Could you check a few things on this model? Use its own coordinates, in mm. Face numbers are marked on the shaded views. A direction names the side the tool comes from. Give positions to 0.01 mm unless a question says otherwise; leave off trailing zeros. Loops run counter-clockwise (first coordinate to the right, second up) from the corner with the lowest first, then second, coordinate; pieces in that order, holes last. Notation, with made-up numbers: M -37,69 L 2,69 A28 ccw 2,91 Z; hole C -3,55 d11. An arc over 180 degrees is marked long. Use a Markdown table: item, result. Add a question column.
1) If I drill on line 1 along Y through (x, z) = (15.25, 3.5); line 2 along Y through (x, z) = (-14.15, 3.5); line 3 along Z through (x, y) = (-14.75, 5.5), over which ranges is the centre line in solid material (lowest first)? Write a range as [from, to].
2) Which directions (+Z, -Z, +X, -X, +Y, -Y) give clear straight access to the entire face, cutting with the end or side of a thin tool? Please do the marked faces 4, 5 and 6.
3) Suppose I cut it at A-A on x = 7. List the corners of the cut face in (y, z) for me, and give its area (3 significant figures).
4) We'd pull the mould along Y, two halves only. Please class the marked faces 1, 2 and 3: +Y half, -Y half, draft (parallel to the pull), parting line (faces both ways), or undercut.
5) Will these pins go through, and if not, where does the flat tip stop? pin 1 Ø1.8 at (y, z) = (-5.5, 3.5) entering from +X; pin 2 Ø3 at (x, y) = (-14.5, -4.5) entering from +Z; pin 3 Ø1.5 at (x, z) = (12.5, 5) entering from -Y.
6) Suppose I cut it at B-B on z = 5.5. List the corners of the cut face in (x, y) for me.
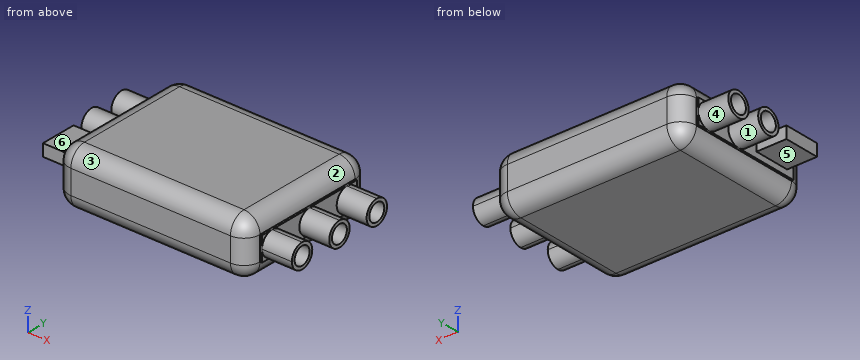
```python
from build123d import *

# Parameters (mm, degrees)
F1_DEPTH  = 7
F2_R      = 2
F3_R      = 1.1
F4_DEPTH  = 4
F5_R      = 1.5
F5_R_2    = 1.1
F6_DEPTH  = 4
F5_W      = 4.5
F5_H      = 1.5
F7_W      = 14
F7_H      = 3
F8_DEPTH  = 0.25
F9_W      = 14
F9_H      = 3
F10_DEPTH = 0.25


with BuildPart() as f1:
    # F0 (on Top) → F1 (new body)
    with BuildSketch(Plane.XY):
        with BuildLine():
            ThreePointArc((12, 7), (11.4142135624, 8.4142135624), (10, 9))
            Line((10, 9), (-10, 9))
            ThreePointArc((-10, 9), (-11.4142135624, 8.4142135624), (-12, 7))
            Line((-12, 7), (-12, -7))
            ThreePointArc((-12, -7), (-11.4142135624, -8.4142135624), (-10, -9))
            Line((-10, -9), (10, -9))
            ThreePointArc((10, -9), (11.4142135624, -8.4142135624), (12, -7))
            Line((12, -7), (12, 7))
        make_face()
    extrude(amount=F1_DEPTH)

    # F2
    f2_edges = [f1.edges().sort_by_distance(p)[0] for p in [
        (11.414214, 8.414214, 7),
        (0, 9, 7),
        (-11.414214, 8.414214, 7),
        (-12, 0, 7),
        (-11.414214, -8.414214, 7),
        (0, -9, 7),
        (11.414214, -8.414214, 7),
        (12, 0, 7),
        (11.414214, 8.414214, 0),
        (0, 9, 0),
        (-11.414214, 8.414214, 0),
        (-12, 0, 0),
        (-11.414214, -8.414214, 0),
        (0, -9, 0),
        (11.414214, -8.414214, 0),
        (12, 0, 0),
    ]]
    fillet(f2_edges, radius=F2_R)



with BuildPart() as f4:
    # F3 (on face) → F4 (new body)
    with BuildSketch(Plane.YZ.offset(12)):
        with BuildLine():
            ThreePointArc((-4, 3.5), (-4.4393398246, 4.5606601681), (-5.4999999897, 5))
            ThreePointArc((-5.4999999897, 5), (-6.5606601681, 4.5606601754), (-7, 3.5))
            ThreePointArc((-7, 3.5), (-6.5606601718, 2.4393398282), (-5.5, 2))
            ThreePointArc((-5.5, 2), (-4.4393398282, 2.4393398282), (-4, 3.5))
        make_face()
        with Locations((-5.5, 3.5)):
            Circle(F3_R, mode=Mode.SUBTRACT)
    extrude(amount=F4_DEPTH)


with BuildPart() as f4b:
    # F3 (on face) → F4, piece 2 (new body)
    with BuildSketch(Plane.YZ.offset(12)):
        with BuildLine():
            ThreePointArc((0, 2), (1.0606601718, 2.4393398282), (1.5, 3.5))
            ThreePointArc((1.5, 3.5), (1.0606601718, 4.5606601718), (0, 5))
            ThreePointArc((0, 5), (-1.5, 3.5), (0, 2))
        make_face()
        with Locations((0, 3.5)):
            Circle(F3_R, mode=Mode.SUBTRACT)
    extrude(amount=F4_DEPTH)


with BuildPart() as f4c:
    # F3 (on face) → F4, piece 3 (new body)
    with BuildSketch(Plane.YZ.offset(12)):
        with BuildLine():
            ThreePointArc((7, 3.5), (6.5606601718, 4.5606601718), (5.5, 5))
            ThreePointArc((5.5, 5), (4, 3.499999998), (5.5000000039, 2))
            ThreePointArc((5.5000000039, 2), (6.5606601732, 2.4393398296), (7, 3.5))
        make_face()
        with Locations((5.5, 3.5)):
            Circle(F3_R, mode=Mode.SUBTRACT)
    extrude(amount=F4_DEPTH)


with BuildPart() as f6:
    # F5 (on face) → F6 (new body)
    with BuildSketch(Plane(origin=(-12, 0, 0), x_dir=(0, -1, 0), z_dir=(-1, 0, 0))):
        with Locations((-5.5, 3.5)):
            Circle(F5_R)
        with Locations((-5.5, 3.5)):
            Circle(F5_R_2, mode=Mode.SUBTRACT)
    extrude(amount=F6_DEPTH)


with BuildPart() as f6b:
    # F5 (on face) → F6, piece 2 (new body)
    with BuildSketch(Plane(origin=(-12, 0, 0), x_dir=(0, -1, 0), z_dir=(-1, 0, 0))):
        with Locations((-1.1, 3.5)):
            Circle(F5_R)
        with Locations((-1.1, 3.5)):
            Circle(F5_R_2, mode=Mode.SUBTRACT)
    extrude(amount=F6_DEPTH)


with BuildPart() as f6c:
    # F5 (on face) → F6, piece 3 (new body)
    with BuildSketch(Plane(origin=(-12, 0, 0), x_dir=(0, -1, 0), z_dir=(-1, 0, 0))):
        with Locations((3.8085386623, 3.5)):
            Rectangle(F5_W, F5_H)
    extrude(amount=F6_DEPTH)


with BuildPart() as f1_1:
    add(f1.part)

    add(f4.part)  # F8 merges F4

    add(f4b.part)  # F8 merges F4b

    add(f4c.part)  # F8 merges F4c
    # F7 (on face) → F8 (join)
    with BuildSketch(Plane.YZ.offset(12)):
        with Locations((0, 3.5)):
            Rectangle(F7_W, F7_H)
    extrude(amount=F8_DEPTH)


    add(f6.part)  # F10 merges F6

    add(f6b.part)  # F10 merges F6b

    add(f6c.part)  # F10 merges F6c
    # F9 (on face) → F10 (join)
    with BuildSketch(Plane(origin=(-12, 0, 0), x_dir=(0, -1, 0), z_dir=(-1, 0, 0))):
        with Locations((0, 3.5)):
            Rectangle(F9_W, F9_H)
    extrude(amount=F10_DEPTH)


solid = f1_1.part
```
Answer block:
| question | item | result |
|---|---|---|
| 1 | line 1 | y = [-7, -6.6], [-4.4, -4], [-1.5, -1.1], [1.1, 1.5], [4, 4.4], [6.6, 7] |
| 1 | line 2 | y = [-6.06, -1.56], [-0.4, 0], [2.2, 2.6], [4, 4.4], [6.6, 7] |
| 1 | line 3 | z = [2, 2.4], [4.6, 5] |
| 2 | face 4 | -X |
| 2 | face 5 | -Z, -X, -Y |
| 2 | face 6 | +Z, -X, -Y |
| 3 | outline | M -9,2 A2 ccw -7,0 L 7,0 A2 ccw 9,2 L 9,5 A2 ccw 7,7 L -7,7 A2 ccw -9,5 Z |
| 3 | area | 123 mm^2 |
| 4 | face 1 | undercut |
| 4 | face 2 | draft |
| 4 | face 3 | -Y half |
| 5 | pin 1 | stops at x = 12.25 |
| 5 | pin 2 | stops at z = 4.25 |
| 5 | pin 3 | stops at y = -7.97 |
| 6 | outline | M -11.94,-7 A1.94 ccw -10,-8.94 L 10,-8.94 A1.94 ccw 11.94,-7 L 11.94,7 A1.94 ccw 10,8.94 L -10,8.94 A1.94 ccw -11.94,7 Z |
